from build123d import *

# Parameters (mm, degrees)
F0_W     = 68
F0_H     = 5
F0_R     = 5
F0_W_2   = 5
F0_H_2   = 48
F1_DEPTH = 5


with BuildPart() as f1:
    # F0 (on Top) → F1 (new body)
    with BuildSketch(Plane.XY):
        with Locations((136, -122.5)):
            Rectangle(F0_W, F0_H)
        Polygon((102, -120), (170, -120), (170, -72), (170, -24), (170, 24), (170, 72), (170, 120), (102, 120), (34, 120), (-34, 120), (-102, 120), (-170, 120), (-170, 72), (-170, 24), (-170, -24), (-170, -72), (-170, -120), (-102, -120), (-34, -120), (34, -120), align=None)
        with Locations((-140, -95)):
            Circle(F0_R, mode=Mode.SUBTRACT)
        with Locations((-85, -95)):
            Circle(F0_R, mode=Mode.SUBTRACT)
        with Locations((-30, -95)):
            Circle(F0_R, mode=Mode.SUBTRACT)
        with Locations((-140, -47)):
            Circle(F0_R, mode=Mode.SUBTRACT)
        with Locations((-85, -47)):
            Circle(F0_R, mode=Mode.SUBTRACT)
        with Locations((-30, -47)):
            Circle(F0_R, mode=Mode.SUBTRACT)
        with Locations((25, -95)):
            Circle(F0_R, mode=Mode.SUBTRACT)
        with Locations((80, -95)):
            Circle(F0_R, mode=Mode.SUBTRACT)
        with Locations((135, -95)):
            Circle(F0_R, mode=Mode.SUBTRACT)
        with Locations((25, -47)):
            Circle(F0_R, mode=Mode.SUBTRACT)
        with Locations((80, -47)):
            Circle(F0_R, mode=Mode.SUBTRACT)
        with Locations((135, -47)):
            Circle(F0_R, mode=Mode.SUBTRACT)
        with Locations((-140, 1)):
            Circle(F0_R, mode=Mode.SUBTRACT)
        with Locations((-140, 49)):
            Circle(F0_R, mode=Mode.SUBTRACT)
        with Locations((-85, 1)):
            Circle(F0_R, mode=Mode.SUBTRACT)
        with Locations((-30, 1)):
            Circle(F0_R, mode=Mode.SUBTRACT)
        with Locations((-85, 49)):
            Circle(F0_R, mode=Mode.SUBTRACT)
        with Locations((-30, 49)):
            Circle(F0_R, mode=Mode.SUBTRACT)
        with Locations((-140, 97)):
            Circle(F0_R, mode=Mode.SUBTRACT)
        with Locations((-85, 97)):
            Circle(F0_R, mode=Mode.SUBTRACT)
        with Locations((-30, 97)):
            Circle(F0_R, mode=Mode.SUBTRACT)
        with Locations((25, 1)):
            Circle(F0_R, mode=Mode.SUBTRACT)
        with Locations((80, 1)):
            Circle(F0_R, mode=Mode.SUBTRACT)
        with Locations((25, 49)):
            Circle(F0_R, mode=Mode.SUBTRACT)
        with Locations((80, 49)):
            Circle(F0_R, mode=Mode.SUBTRACT)
        with Locations((135, 1)):
            Circle(F0_R, mode=Mode.SUBTRACT)
        with Locations((135, 49)):
            Circle(F0_R, mode=Mode.SUBTRACT)
        with Locations((25, 97)):
            Circle(F0_R, mode=Mode.SUBTRACT)
        with Locations((80, 97)):
            Circle(F0_R, mode=Mode.SUBTRACT)
        with Locations((135, 97)):
            Circle(F0_R, mode=Mode.SUBTRACT)
        with Locations((172.5, -48)):
            Rectangle(F0_W_2, F0_H_2)
        with Locations((0, -122.5)):
            Rectangle(F0_W, F0_H)
        with Locations((172.5, 48)):
            Rectangle(F0_W_2, F0_H_2)
        with Locations((-136, -122.5)):
            Rectangle(F0_W, F0_H)
        with Locations((136, 122.5)):
            Rectangle(F0_W, F0_H)
        with Locations((-172.5, -48)):
            Rectangle(F0_W_2, F0_H_2)
        with Locations((0, 122.5)):
            Rectangle(F0_W, F0_H)
        with Locations((-172.5, 48)):
            Rectangle(F0_W_2, F0_H_2)
        with Locations((-136, 122.5)):
            Rectangle(F0_W, F0_H)
    extrude(amount=F1_DEPTH)


solid = f1.part
Geometry: final body of the model. Coordinates: model frame, mm. Give positions to 0.01 mm unless a question says otherwise; leave off trailing zeros. Order: outer loops, then holes, each group sorted by start corner. A loop starts at its lowest first (then second) coordinate and runs counter-clockwise, first axis right, second up. Notation, with made-up numbers: (-24, -12.75) - (-7, -12.75) arc R27 ccw to (-7, 3.25) - close; hole circle Ø1 at (-14, -31). An arc over 180 degrees is marked (long way). Use CSV: the item, a comma, the result in double quotes.
1. Section query D-D (y = 97). Output: boundary loops of the cut face in (x, z).
Answers below:
outline,"(-170, 0) - (-145, 0) - (-145, 5) - (-170, 5) - close; (-135, 0) - (-90, 0) - (-90, 5) - (-135, 5) - close; (-80, 0) - (-35, 0) - (-35, 5) - (-80, 5) - close; (-25, 0) - (20, 0) - (20, 5) - (-25, 5) - close; (30, 0) - (75, 0) - (75, 5) - (30, 5) - close; (85, 0) - (130, 0) - (130, 5) - (85, 5) - close; (140, 0) - (170, 0) - (170, 5) - (140, 5) - close"
2. Section query C-C (z = 0.85). Give the number of separate pieces and of enclosed holes in the cut face, plus the area to 3 significant figures.
Answers below:
separate pieces,"1"
enclosed holes,"30"
area,"82,200 mm2"
3. Section query B-B (x = -140). Output: boundary loops of the cut face in (y, z), plus the area to 3 significant figures.
Answers below:
outline,"(-125, 0) - (-100, 0) - (-100, 5) - (-125, 5) - close; (-90, 0) - (-52, 0) - (-52, 5) - (-90, 5) - close; (-42, 0) - (-4, 0) - (-4, 5) - (-42, 5) - close; (6, 0) - (44, 0) - (44, 5) - (6, 5) - close; (54, 0) - (92, 0) - (92, 5) - (54, 5) - close; (102, 0) - (125, 0) - (125, 5) - (102, 5) - close"
area,"1,000 mm2"
4. Contact query for flat-ended pins moving along their axis: pin 1 (3 mm diameter, centred on x = 23, y = -54, fed in from -Z); pin 2 (2.5 mm diameter, centred on y = 122, z = 3.5, fed in from -X); pin 3 (6 mm diameter, centred on x = 80, y = 97, fed in from +Z). Output: stop coordinate, or through.
Answers below:
pin 1,"z = 0"
pin 2,"x = -170"
pin 3,"through"
5. Mould query, pull axis X, two halves, no side actions, for faces 1 (the face through (24.349, -42.043, 2.465)), 2 (the face through (-2, 2, 5)). Classes: +X half, -X half, draft (parallel to the pull), parting line (faces both ways), or undercut.
Answers below:
face 1,"undercut"
face 2,"draft"
6. Material intervals for line 1 along Y through (x, z) = (25, 1.8); line 2 along Y through (x, z) = (80, 1.75); line 3 along Y through (x, z) = (44.5, 1.05), sorted ascending. Write a range as from..to.
Answers below:
line 1,"-125..-100, -90..-52, -42..-4, 6..44, 54..92, 102..125"
line 2,"-120..-100, -90..-52, -42..-4, 6..44, 54..92, 102..120"
line 3,"-120..120"
7. Section query A-A (y = 49). Output: boundary loops of the cut face in (x, z), plus the area to 3 significant figures.
Answers below:
outline,"(-175, 0) - (-145, 0) - (-145, 5) - (-175, 5) - close; (-135, 0) - (-90, 0) - (-90, 5) - (-135, 5) - close; (-80, 0) - (-35, 0) - (-35, 5) - (-80, 5) - close; (-25, 0) - (20, 0) - (20, 5) - (-25, 5) - close; (30, 0) - (75, 0) - (75, 5) - (30, 5) - close; (85, 0) - (130, 0) - (130, 5) - (85, 5) - close; (140, 0) - (175, 0) - (175, 5) - (140, 5) - close"
area,"1,450 mm2"
